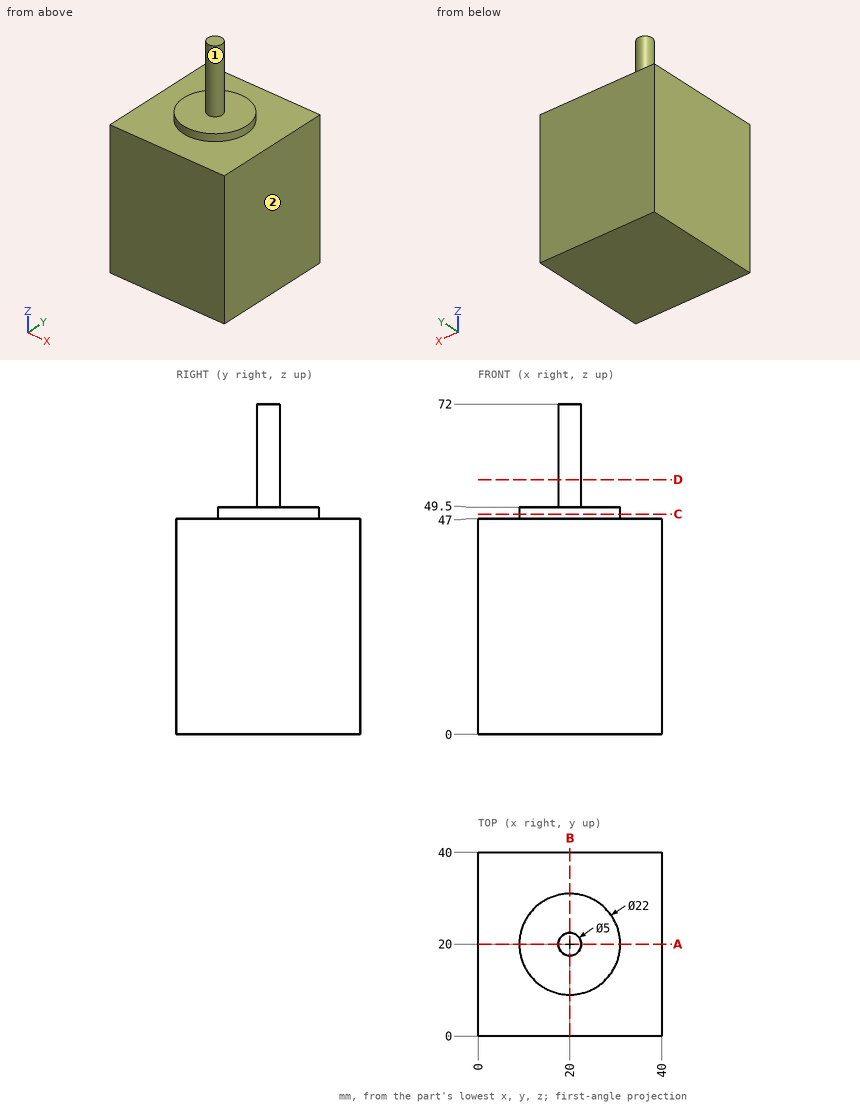
The figure shows three views and two pictorial views of one solid part (mm, origin at its lowest corner). Answer the questions. A direction names the side the tool comes from. Round coordinates to 2 decimals unless told otherwise and drop trailing zeros. Write each loop counter-clockwise with the first axis right and the second up, starting at its lowest first coordinate (ties: lowest second). Pieces come first, ordered by that corner, then holes. Notation, with made-up numbers: (14.5, 9) - (24.5, 9) arc R10 ccw to (24.5, 22) - close; hole circle Ø5 at (85, -37.5). An arc over 180 degrees is marked (long way). Answer in a Markdown table with one row per item. Add a question column.
1. A cutting plane is placed at D-D, the plane z = 55.5. Determine the outline of the cut face in (x, y).
2. Find the intervals of material crossed by line 1 along Z through (x, y) = (19.5, 30.5); line 2 along Z through (x, y) = (38, 25.5); line 3 along Y through (x, z) = (20, 68.5), in increasing order. Write a range as from..to.
3. Given pin 1 (12 mm diameter, centred on x = 25.5, y = 4.5, fed in from +Z), flat-ended and moving along its own axis, determine where the tip first touches the part or whether it passes through.
4. For the marked faces 1 and 2, determine the directions among +Z, -Z, +X, -X, +Y, -Y from which every point of the face is accessible in a straight line to the end or side of a thin tool.
5. A cutting plane is placed at A-A, the plane y = 20. Determine the outline of the cut face in (x, z).
6. A cutting plane is placed at C-C, the plane z = 48. Determine the outline of the cut face in (x, y), and give its area (3 significant figures).
Worked out:
| question | item | result |
|---|---|---|
| 1 | outline | circle Ø5 at (20, 20) |
| 2 | line 1 | 0..49.5 |
| 2 | line 2 | 0..47 |
| 2 | line 3 | 17.5..22.5 |
| 3 | pin 1 | z = 49.5 |
| 4 | face 1 | +Z |
| 4 | face 2 | +Z, -Z, +X, +Y, -Y |
| 5 | outline | (0, 0) - (40, 0) - (40, 47) - (31, 47) - (31, 49.5) - (22.5, 49.5) - (22.5, 72) - (17.5, 72) - (17.5, 49.5) - (9, 49.5) - (9, 47) - (0, 47) - close |
| 6 | outline | circle Ø22 at (20, 20) |
| 6 | area | 380 mm^2 |
